from build123d import *

# Parameters (mm, degrees)
EXTRUDE_1_DEPTH     = 30
SKETCH_2_R          = 3.05
CUT_EXTRUDE_1_DEPTH = 30
SKETCH_3_R          = 3.05
CUT_EXTRUDE_2_DEPTH = 30
CUT_EXTRUDE_3_DEPTH = 54


with BuildPart() as part:
    # 草图1 → 凸台-拉伸1 (new body)
    with BuildSketch(Plane.XY):
        Polygon((-13, -20.797836643), (-13, -73.797836643), (13, -73.797836643), (13, -20.797836643), (15, -20.797836643), (15, -75.797836643), (-15, -75.797836643), (-15, -20.797836643), align=None)
    extrude(amount=EXTRUDE_1_DEPTH)

    # 草图2 → 切除-拉伸1 (cut)
    with BuildSketch(Plane.XZ.offset(75.797836643)):
        with Locations((0, 15)):
            Circle(SKETCH_2_R)
    extrude(amount=-CUT_EXTRUDE_1_DEPTH, mode=Mode.SUBTRACT)

    # 草图3 → 切除-拉伸2 (cut)
    with BuildSketch(Plane(origin=(15, 0, 0), x_dir=(0, 0, -1), z_dir=(1, 0, 0))):
        with Locations((-15, -30.797836643)):
            Circle(SKETCH_3_R)
    extrude(amount=-CUT_EXTRUDE_2_DEPTH, mode=Mode.SUBTRACT)

    # 草图4 → 切除-拉伸3 (cut)
    with BuildSketch(Plane.ZY.offset(15)):
        with BuildLine():
            Line((0, -73.797836643), (7.608366664, -29.527499433))
            ThreePointArc((7.608366664, -29.527499433), (15, -23.297836643), (22.391633336, -29.527499433))
            Line((22.391633336, -29.527499433), (30, -73.797836643))
            Line((30, -73.797836643), (30, -20.797836643))
            Line((30, -20.797836643), (0, -20.797836643))
            Line((0, -20.797836643), (0, -73.797836643))
        make_face()
    extrude(amount=-CUT_EXTRUDE_3_DEPTH, mode=Mode.SUBTRACT)


solid = part.part
Input: part model. Units: mm. Frame: model coordinates. A direction names the side the tool comes from. Coordinates: 2 decimals unless noted, no trailing zeros. Order: outer loops, then holes, each group sorted by start corner. A loop starts at its lowest first (then second) coordinate and runs counter-clockwise, first axis right, second up. Notation, with made-up numbers: M -36,42 L 2,42 A6 ccw 2,49 Z; hole C 87,-31 d11. An arc over 180 degrees is marked long. Answer in a Markdown table with one row per item.
(1) Draft query along X for faces 1 (the cylindrical face through (-0.397, -74.812, 18.024)), 2 (the flat face through (15, -55, 15)), 3 (the cylindrical face through (14.014, -33.775, 15.661)). Return one class per face: pulls with the +X half, pulls with the -X half, needs draft (parallel to the pull), parting line crosses it, or undercut.
Numbers:
| item | result |
|---|---|
| face 1 | undercut |
| face 2 | pulls with the +X half |
| face 3 | needs draft |
(2) Contact query for flat-ended pins moving along their axis: pin 1 Ø8 at (x, z) = (3.5, 14) entering from +Y; pin 2 Ø1.5 at (y, z) = (-32, 15.5) entering from +X; pin 3 Ø8 at (y, z) = (-30.8, 15) entering from -X. Output: stop coordinate, or through.
Numbers:
| item | result |
|---|---|
| pin 1 | stops at y = -73.8 |
| pin 2 | passes through |
| pin 3 | stops at x = -15 |
(3) Section query A-A, the plane x = 0. Output: boundary loops of the cut face in (y, z).
Numbers:
| item | result |
|---|---|
| outline | M -75.8,0 L -73.8,0 L -73.8,11.95 L -75.8,11.95 Z; M -75.8,18.05 L -73.8,18.05 L -73.8,30 L -75.8,30 Z |
(4) Section query C-C, the plane y = -31.5. Output: boundary loops of the cut face in (x, z).
Numbers:
| item | result |
|---|---|
| outline | M -15,7.27 L -13,7.27 L -13,12.03 L -15,12.03 Z; M -15,17.97 L -13,17.97 L -13,22.73 L -15,22.73 Z; M 13,7.27 L 15,7.27 L 15,12.03 L 13,12.03 Z; M 13,17.97 L 15,17.97 L 15,22.73 L 13,22.73 Z |
(5) Material intervals for line 1 (X direction, y = -50.5, z = 8.25); line 2 (Y direction, x = -14.35, z = 15); line 3 (Z direction, x = 0, y = -75.3), sorted ascending. Write a range as [from, to].
Numbers:
| item | result |
|---|---|
| line 1 | x = [-15, -13], [13, 15] |
| line 2 | y = [-75.8, -33.85], [-27.75, -23.3] |
| line 3 | z = [0, 11.95], [18.05, 30] |
(6) Section query D-D, the plane z = 26.5. Output: boundary loops of the cut face in (x, y).
Numbers:
| item | result |
|---|---|
| outline | M -15,-75.8 L 15,-75.8 L 15,-53.43 L 13,-53.43 L 13,-73.8 L -13,-73.8 L -13,-53.43 L -15,-53.43 Z |
(7) Access query for faces 4 (the flat face through (-15, -56, 15)), 5 (the flat face through (-13, -54, 15)). Directions: +Z, -Z, +X, -X, +Y, -Y. A direction counts if a zero-diameter tool reaches every point of the face in a straight line with its end or side. Return the directions, or none.
Numbers:
| item | result |
|---|---|
| face 4 | +Z, -Z, -X, +Y, -Y |
| face 5 | +Z, -Z, +Y |
(8) Section query B-B, the plane y = -57. Output: boundary loops of the cut face in (x, z), plus the area to 3 significant figures.
Numbers:
| item | result |
|---|---|
| outline | M -15,2.89 L -13,2.89 L -13,27.11 L -15,27.11 Z; M 13,2.89 L 15,2.89 L 15,27.11 L 13,27.11 Z |
| area | 96.9 mm^2 |
